from build123d import *

# Parameters (mm, degrees)
SKETCH_1_R      = 2.5
SKETCH_1_R_2    = 11
SKETCH_1_R_3    = 2
SKETCH_1_R_4    = 1.5
SKETCH_1_R_5    = 6
SKETCH_1_W      = 8.2
SKETCH_1_H      = 124
EXTRUDE_1_DEPTH = 5


with BuildPart() as part:
    # 草图1 → 凸台-拉伸1 (new body)
    with BuildSketch(Plane(origin=(0, 0, 0), x_dir=(1, 0, 0), z_dir=(0, 1, 0))):
        with BuildLine():
            Line((-235, 92.5), (235, 92.5))
            Line((235, 92.5), (235, -92.5))
            Line((235, -92.5), (104, -92.5))
            Line((104, -92.5), (82, -92.5))
            ThreePointArc((82, -92.5), (0, -80.151224636), (-82, -92.5))
            Line((-82, -92.5), (-104, -92.5))
            Line((-104, -92.5), (-235, -92.5))
            Line((-235, -92.5), (-235, 92.5))
        make_face()
        with Locations((-104, 37.5)):
            Circle(SKETCH_1_R, mode=Mode.SUBTRACT)
        with Locations((-104, -44.5)):
            Circle(SKETCH_1_R, mode=Mode.SUBTRACT)
        with Locations((104, 37.5)):
            Circle(SKETCH_1_R, mode=Mode.SUBTRACT)
        with Locations((104, -44.5)):
            Circle(SKETCH_1_R, mode=Mode.SUBTRACT)
        with Locations((-74, 57.5)):
            Circle(SKETCH_1_R_2, mode=Mode.SUBTRACT)
        with Locations((-26.67, 57.5)):
            Circle(SKETCH_1_R_2, mode=Mode.SUBTRACT)
        with Locations((20.67, 57.5)):
            Circle(SKETCH_1_R_2, mode=Mode.SUBTRACT)
        with Locations((68, 57.5)):
            Circle(SKETCH_1_R_2, mode=Mode.SUBTRACT)
        with Locations((64, -44.5)):
            Circle(SKETCH_1_R_2, mode=Mode.SUBTRACT)
        with Locations((-204, 57.5)):
            Circle(SKETCH_1_R_2, mode=Mode.SUBTRACT)
        with Locations((-74, -44.5)):
            Circle(SKETCH_1_R_2, mode=Mode.SUBTRACT)
        with Locations((149, 0)):
            Circle(SKETCH_1_R_3, mode=Mode.SUBTRACT)
        with Locations((193, 0)):
            Circle(SKETCH_1_R_3, mode=Mode.SUBTRACT)
        with Locations((149, 45)):
            Circle(SKETCH_1_R_3, mode=Mode.SUBTRACT)
        with Locations((149, -45)):
            Circle(SKETCH_1_R_3, mode=Mode.SUBTRACT)
        with Locations((193, 45)):
            Circle(SKETCH_1_R_3, mode=Mode.SUBTRACT)
        with Locations((193, -45)):
            Circle(SKETCH_1_R_3, mode=Mode.SUBTRACT)
        with Locations((-124, -74)):
            Circle(SKETCH_1_R_4, mode=Mode.SUBTRACT)
        with Locations((-124, 8.5)):
            Circle(SKETCH_1_R_4, mode=Mode.SUBTRACT)
        with Locations((-215, -74)):
            Circle(SKETCH_1_R_4, mode=Mode.SUBTRACT)
        with Locations((-215, 16)):
            Circle(SKETCH_1_R_4, mode=Mode.SUBTRACT)
        with Locations((-144, 57.5)):
            Circle(SKETCH_1_R_5, mode=Mode.SUBTRACT)
        with Locations((0, -70.101989155)):
            Circle(SKETCH_1_R_3, mode=Mode.SUBTRACT)
        with Locations((-174, -82.5)):
            Circle(SKETCH_1_R_3, mode=Mode.SUBTRACT)
        with Locations((174, -82.5)):
            Circle(SKETCH_1_R_3, mode=Mode.SUBTRACT)
        with Locations((-225, 0)):
            Circle(SKETCH_1_R_3, mode=Mode.SUBTRACT)
        with Locations((225, 0)):
            Circle(SKETCH_1_R_3, mode=Mode.SUBTRACT)
        with Locations((173, 0)):
            Rectangle(SKETCH_1_W, SKETCH_1_H, mode=Mode.SUBTRACT)
    extrude(amount=EXTRUDE_1_DEPTH)


solid = part.part
The model under review builds one solid part; all positions refer to its coordinate system, in mm. Give positions to 0.01 mm unless a question says otherwise; leave off trailing zeros. Order: outer loops, then holes, each group sorted by start corner. A loop starts at its lowest first (then second) coordinate and runs counter-clockwise, first axis right, second up. Notation, with made-up numbers: M -20,20.5 L -3,20.5 A13 cw -3,40.5 Z; hole C 69.25,48 d1. An arc over 180 degrees is marked long. Answer in a Markdown table with one row per item. Add a question column.
1. For pin 1 Ø17.5 at (x, z) = (64, 44.5) entering from +Y; pin 2 Ø3 at (x, y) = (65.5, 3) entering from +Z, all flat-tipped, find the tip position at first contact; note any pin that passes through.
2. Add section A-A on x = -204. State the section outline as (y, z) points, plus the area to 3 significant figures.
3. To check wall thickness, follow line 1 along X through (y, z) = (2.2, 74); line 2 along Z through (x, y) = (193, 2.85); line 3 along X through (y, z) = (0.35, -45). State the ranges of each line that lie inside material, in increasing order.
4. Add section D-D on x = -53.5. State the section outline as (y, z) points.
5. Mouldability with a two-part tool opening along Z and no side actions: class faces 1 (the cylindrical face through (-148.76, 2.46, -53.85)), 2 (the cylindrical face through (1.165, 2.465, 80.154)), 3 (the flat face through (3, 5, -1)) as released by +Z, released by -Z, zero draft, split by the parting line, or undercut.
6. Add section B-B on z = 19.5. State the section outline as (x, y) points, plus the area to 3 significant figures.
7. Add section C-C on y = 3.35. Count the separate pieces of the cut face and the enclosed holes in it, plus the area to 3 significant figures.
The answers:
| question | item | result |
|---|---|---|
| 1 | pin 1 | through |
| 1 | pin 2 | z = 88.33 |
| 2 | outline | M 0,-92.5 L 5,-92.5 L 5,-68.5 L 0,-68.5 Z; M 0,-46.5 L 5,-46.5 L 5,92.5 L 0,92.5 Z |
| 2 | area | 815 mm2 |
| 3 | line 1 | -235 to -216.5, -213.5 to -125.5, -122.5 to 235 |
| 3 | line 2 | -92.5 to -47, -43 to -2, 2 to 43, 47 to 92.5 |
| 3 | line 3 | -235 to 147, 151 to 168.9, 177.1 to 191, 195 to 235 |
| 4 | outline | M 0,-92.5 L 5,-92.5 L 5,85.34 L 0,85.34 Z |
| 5 | face 1 | undercut |
| 5 | face 2 | released by +Z |
| 5 | face 3 | zero draft |
| 6 | outline | M -235,0 L 168.9,0 L 168.9,5 L -235,5 Z; M 177.1,0 L 235,0 L 235,5 L 177.1,5 Z |
| 6 | area | 2,310 mm2 |
| 7 | separate pieces | 1 |
| 7 | enclosed holes | 28 |
| 7 | area | 81,600 mm2 |
